Design review of the part built by this model. Coordinates are the model's own, in mm. A direction names the side the tool comes from. Coordinates: 2 decimals unless noted, no trailing zeros. Write each loop counter-clockwise with the first axis right and the second up, starting at its lowest first coordinate (ties: lowest second). Pieces come first, ordered by that corner, then holes. Notation, with made-up numbers: M -26,82.5 L 17,82.5 A8 ccw 17,96.5 Z; hole C 84.25,66 d10. An arc over 180 degrees is marked long. Return JSON: item names as keys, results as strings. Group by question number.
```python
from build123d import *

# Parameters (mm, degrees)
SKETCH1_R           = 3.429
BOSS_EXTRUDE1_DEPTH = 3.175
SKETCH3_R           = 67.945
CUT_EXTRUDE2_DEPTH  = 1.905


with BuildPart() as part:
    # Sketch1 → Boss-Extrude1 (new body)
    with BuildSketch(Plane.XY):
        Polygon((38.1, -79.375), (193.675, -79.375), (193.675, 79.375), (-193.675, 79.375), (-193.675, -79.375), (-38.1, -79.375), (-38.1, -44.323), (38.1, -44.323), align=None)
        with Locations((-177.8, 63.5)):
            Circle(SKETCH1_R, mode=Mode.SUBTRACT)
        with Locations((177.8, 63.5)):
            Circle(SKETCH1_R, mode=Mode.SUBTRACT)
        with Locations((177.8, -63.5)):
            Circle(SKETCH1_R, mode=Mode.SUBTRACT)
        with Locations((-177.8, -63.5)):
            Circle(SKETCH1_R, mode=Mode.SUBTRACT)
    extrude(amount=BOSS_EXTRUDE1_DEPTH)

    # Sketch3 → Cut-Extrude2 (cut)
    with BuildSketch(Plane(origin=(0, 0, 0), x_dir=(-1, 0, 0), z_dir=(0, 0, -1))):
        with Locations((0, 34.925)):
            Circle(SKETCH3_R)
    extrude(amount=-CUT_EXTRUDE2_DEPTH, mode=Mode.SUBTRACT)


solid = part.part
```
Item 1: Add section C-C (z = 0.65). Write out the cut boundary in (x, y) (3 decimals), plus the area to 3 significant figures.
Item 2: Add section B-B (y = -63.5). Write out the cut boundary in (x, z) (3 decimals), plus the area to 3 significant figures.
Item 3: Add section A-A (x = -177.8). Write out the cut boundary in (y, z) (3 decimals).
Item 4: For line 1 (Y direction, x = -177.8, z = 1.5) (3 decimals); line 2 (X direction, y = -47.5, z = 0.55) (3 decimals); line 3 (Z direction, x = -55.5, y = 67) (3 decimals), list the stretches that pass through material, from the lowest coordinate up.
Item 5: The part is to be moulded in two halves that separate along X. For faces 3 (the flat face through (-3, 1, 3.175)), 4 (the cylindrical face through (181.07, -62.47, 1.57)), say which applies: pulls with the +X half, pulls with the -X half, needs draft (parallel to the pull), parting line crosses it, or undercut.
Item 6: For pin 1 (6 mm diameter, centred on x = -177.8, y = -63.5, fed in from -Z), flat-tipped, find the tip position at first contact; note if it passes through.
Item 7: Add section D-D (x = 0). Write out the cut boundary in (y, z) (3 decimals).
Item 8: Machinability: for faces 1 (the cylindrical face through (2.172, -32.985, 0.939)), 2 (the cylindrical face through (181.07, 64.53, 1.57)), which of the approach directions +Z, -Z, +X, -X, +Y, -Y give a long, thin tool a straight path to every point of the face, cutting with its end or side? Answer none if there is none.
Geometry check:
{
 "1": {"outline": "M -193.675,-79.375 L -38.1,-79.375 L -38.1,-44.323 L 38.1,-44.323 L 38.1,-79.375 L 193.675,-79.375 L 193.675,79.375 L 51.388,79.375 A67.945 cw long -51.388,79.375 L -193.675,79.375 Z; hole C -177.8,-63.5 d6.858; hole C -177.8,63.5 d6.858; hole C 177.8,-63.5 d6.858; hole C 177.8,63.5 d6.858", "area": "45,800 mm^2"},
 "2": {"outline": "M -193.675,0 L -181.229,0 L -181.229,3.175 L -193.675,3.175 Z; M -174.371,0 L -38.1,0 L -38.1,3.175 L -174.371,3.175 Z; M 38.1,0 L 174.371,0 L 174.371,3.175 L 38.1,3.175 Z; M 181.229,0 L 193.675,0 L 193.675,3.175 L 181.229,3.175 Z", "area": "944 mm^2"},
 "3": {"outline": "M -79.375,0 L -66.929,0 L -66.929,3.175 L -79.375,3.175 Z; M -60.071,0 L 60.071,0 L 60.071,3.175 L -60.071,3.175 Z; M 66.929,0 L 79.375,0 L 79.375,3.175 L 66.929,3.175 Z"},
 "4": {"line 1": "-79.375 to -66.929, -60.071 to 60.071, 66.929 to 79.375", "line 2": "-193.675 to -38.1, 38.1 to 193.675", "line 3": "1.905 to 3.175"},
 "5": {"face 3": "needs draft", "face 4": "undercut"},
 "6": {"pin 1": "through"},
 "7": {"outline": "M -44.323,0 L -33.02,0 L -33.02,1.905 L 79.375,1.905 L 79.375,3.175 L -44.323,3.175 Z"},
 "8": {"face 1": "-Z", "face 2": "+Z, -Z"}
}
